```python
from build123d import *

# Parameters (mm, degrees)
CROQUIS1_R              = 2
CROQUIS1_R_2            = 1.5
SALIENTE_EXTRUIR1_DEPTH = 2
REDONDEO3_R             = 3


with BuildPart() as part:
    # Croquis1 → Saliente-Extruir1 (new body)
    with BuildSketch(Plane.XY):
        with BuildLine():
            Line((-31.096194078, 38.16726189), (-21.213203436, 28.284271247))
            ThreePointArc((-21.213203436, 28.284271247), (0, 19.497474683), (21.213203436, 28.284271247))
            Line((21.213203436, 28.284271247), (31.096194078, 38.16726189))
            Line((31.096194078, 38.16726189), (38.890872965, 45.961940777))
            Line((38.890872965, 45.961940777), (42.426406871, 42.426406871))
            Line((42.426406871, 42.426406871), (45.961940777, 38.890872965))
            Line((45.961940777, 38.890872965), (38.16726189, 31.096194078))
            Line((38.16726189, 31.096194078), (28.284271247, 21.213203436))
            ThreePointArc((28.284271247, 21.213203436), (19.497474683, 0), (28.284271247, -21.213203436))
            Line((28.284271247, -21.213203436), (38.16726189, -31.096194078))
            Line((38.16726189, -31.096194078), (45.961940777, -38.890872965))
            Line((45.961940777, -38.890872965), (42.426406871, -42.426406871))
            Line((42.426406871, -42.426406871), (38.890872965, -45.961940777))
            Line((38.890872965, -45.961940777), (31.096194078, -38.16726189))
            Line((31.096194078, -38.16726189), (21.213203436, -28.284271247))
            ThreePointArc((21.213203436, -28.284271247), (0, -19.497474683), (-21.213203436, -28.284271247))
            Line((-21.213203436, -28.284271247), (-31.096194078, -38.16726189))
            Line((-31.096194078, -38.16726189), (-38.890872965, -45.961940777))
            Line((-38.890872965, -45.961940777), (-42.426406871, -42.426406871))
            Line((-42.426406871, -42.426406871), (-45.961940777, -38.890872965))
            Line((-45.961940777, -38.890872965), (-38.16726189, -31.096194078))
            Line((-38.16726189, -31.096194078), (-28.284271247, -21.213203436))
            ThreePointArc((-28.284271247, -21.213203436), (-19.497474683, 0), (-28.284271247, 21.213203436))
            Line((-28.284271247, 21.213203436), (-38.16726189, 31.096194078))
            Line((-38.16726189, 31.096194078), (-45.961940777, 38.890872965))
            Line((-45.961940777, 38.890872965), (-42.426406871, 42.426406871))
            Line((-42.426406871, 42.426406871), (-38.890872965, 45.961940777))
            Line((-38.890872965, 45.961940777), (-31.096194078, 38.16726189))
        make_face()
        with Locations((-15.25, 15.25)):
            Circle(CROQUIS1_R, mode=Mode.SUBTRACT)
        with Locations((-24.04163056, 24.04163056)):
            Circle(CROQUIS1_R_2, mode=Mode.SUBTRACT)
        with Locations((-38.890872965, 38.890872965)):
            Circle(CROQUIS1_R_2, mode=Mode.SUBTRACT)
        with Locations(Location((38.890872965, 38.890872965, 0), (0, 0, 180))):
            Circle(CROQUIS1_R_2, mode=Mode.SUBTRACT)
        with Locations(Location((24.04163056, 24.04163056, 0), (0, 0, 180))):
            Circle(CROQUIS1_R_2, mode=Mode.SUBTRACT)
        with Locations(Location((15.25, 15.25, 0), (0, 0, 180))):
            Circle(CROQUIS1_R, mode=Mode.SUBTRACT)
        with Locations((15.25, -15.25)):
            Circle(CROQUIS1_R, mode=Mode.SUBTRACT)
        with Locations((24.04163056, -24.04163056)):
            Circle(CROQUIS1_R_2, mode=Mode.SUBTRACT)
        with Locations((38.890872965, -38.890872965)):
            Circle(CROQUIS1_R_2, mode=Mode.SUBTRACT)
        with Locations(Location((-15.25, -15.25, 0), (0, 0, 180))):
            Circle(CROQUIS1_R, mode=Mode.SUBTRACT)
        with Locations(Location((-24.04163056, -24.04163056, 0), (0, 0, 180))):
            Circle(CROQUIS1_R_2, mode=Mode.SUBTRACT)
        with Locations(Location((-38.890872965, -38.890872965, 0), (0, 0, 180))):
            Circle(CROQUIS1_R_2, mode=Mode.SUBTRACT)
        Circle(CROQUIS1_R_2, mode=Mode.SUBTRACT)
    extrude(amount=SALIENTE_EXTRUIR1_DEPTH)

    # Redondeo3
    redondeo3_edges = [part.edges().sort_by_distance(p)[0] for p in [
        (-38.890872965, 45.961940777, 1),
        (38.890872965, 45.961940777, 1),
        (45.961940777, 38.890872965, 1),
        (45.961940777, -38.890872965, 1),
        (38.890872965, -45.961940777, 1),
        (-38.890872965, -45.961940777, 1),
        (-45.961940777, -38.890872965, 1),
        (-45.961940777, 38.890872965, 1),
    ]]
    fillet(redondeo3_edges, radius=REDONDEO3_R)


solid = part.part
```
Work out the finished part from the listing and answer in its coordinate system (mm). Round coordinates to 2 decimals unless told otherwise and drop trailing zeros. Write each loop counter-clockwise with the first axis right and the second up, starting at its lowest first coordinate (ties: lowest second). Pieces come first, ordered by that corner, then holes.
1) Flat-ended cylindrical pins translate along their axes: P1, Ø5, axis at x = -15.25, y = -15.25, coming from the +Z side; P2, Ø2.5, axis at x = 24.04, y = -24.04, coming from the +Z side. Find the tip coordinate at first contact, or state that the pin passes through.
2) A cutting plane is placed at A-A on y = 15.25. Determine the outline of the cut face in (x, z), and give its area (3 significant figures).
3) Determine the mould class of faces 1 (the face through (-0.3, 19.5, 1)), 2 (the face through (-3, 0, 0)), 3 (the face through (-40.32, -39.34, 0.99)) for opening direction Y: pulls with the +Y half, pulls with the -Y half, needs draft (parallel to the pull), parting line crosses it, or undercut.
4) Consider probe 1 along Y at (x, z) = (0, 1.5); probe 2 along Y at (x, z) = (-15.25, 1); probe 3 along X at (y, z) = (-38.5, 0.85). Determine where each line is inside the solid, lowest interval first.
5) A cutting plane is placed at B-B on x = 35.5. Determine the outline of the cut face in (y, z), and give its area (3 significant figures).
6) A cutting plane is placed at D-D on z = 1.6. Give the number of separate pieces and of enclosed holes in the cut face, and give its area (3 significant figures).
Entries:
1. P1: stops at z = 2
1. P2: passes through
2. outline: (-23.66, 0) - (-17.25, 0) - (-17.25, 2) - (-23.66, 2) - close; (-13.25, 0) - (13.25, 0) - (13.25, 2) - (-13.25, 2) - close; (17.25, 0) - (23.66, 0) - (23.66, 2) - (17.25, 2) - close
2. area: 78.7 mm2
3. face 1: pulls with the +Y half
3. face 2: needs draft
3. face 3: undercut
4. probe 1: y = -19.5 to -1.5, 1.5 to 19.5
4. probe 2: y = -23.66 to -17.25, -13.25 to 13.25, 17.25 to 23.66
4. probe 3: x = -44.69 to -40.34, -37.44 to -31.43, 31.43 to 37.44, 40.34 to 44.69
5. outline: (-42.57, 0) - (-28.43, 0) - (-28.43, 2) - (-42.57, 2) - close; (28.43, 0) - (42.57, 0) - (42.57, 2) - (28.43, 2) - close
5. area: 56.6 mm2
6. separate pieces: 1
6. enclosed holes: 13
6. area: 2,940 mm2
